The listing builds one solid part. Answer for the finished solid, in the listing's coordinates (mm). Round coordinates to 2 decimals unless told otherwise and drop trailing zeros. Order: outer loops, then holes, each group sorted by start corner. A loop starts at its lowest first (then second) coordinate and runs counter-clockwise, first axis right, second up. Notation, with made-up numbers: (37.5, 10) - (72.5, 10) arc R20 cw to (72.5, 33) - close; hole circle Ø1 at (44, -12). An arc over 180 degrees is marked (long way). Write item = value, one per line.
from build123d import *

# Parameters (mm, degrees)
SKETCH1_W                = 62
SKETCH1_H                = 60
BOSS_EXTRUDE1_DEPTH      = 3
F_4_0_4_DIAMETER_HOLE1_D = 4
FILLET1_R                = 5


with BuildPart() as part:
    # Sketch1 → Boss-Extrude1 (new body)
    with BuildSketch(Plane(origin=(0, 0, 0), x_dir=(1, 0, 0), z_dir=(0, 1, 0))):
        Rectangle(SKETCH1_W, SKETCH1_H)
    extrude(amount=BOSS_EXTRUDE1_DEPTH)

    # Ø4.0 (4) Diameter Hole1 (through all)
    with Locations(Plane(origin=(0, 3, 0), x_dir=(1, 0, 0), z_dir=(0, 1, 0))):
        with Locations((-26, 25), (26, -25), (26, 25), (-26, -25)):
            Hole(F_4_0_4_DIAMETER_HOLE1_D / 2)

    # Fillet1
    fillet1_edges = [part.edges().sort_by_distance(p)[0] for p in [
        (31, 1.5, 30),
        (-31, 1.5, 30),
        (-31, 1.5, -30),
        (31, 1.5, -30),
    ]]
    fillet(fillet1_edges, radius=FILLET1_R)


solid = part.part
Q1. Find the intervals of material crossed by line 1 (Z direction, x = 26, y = 1.2); line 2 (X direction, y = 1.85, z = 25); line 3 (X direction, y = 0.15, z = 26), in increasing order. Write a range as from..to.
Model answer:
line_1 = -30..-27, -23..23, 27..30
line_2 = -31..-28, -24..24, 28..31
line_3 = -30.9..-27.73, -24.27..24.27, 27.73..30.9
Q2. Section A-A on y = 2.4 is taken. Determine the outline of the cut face in (x, z).
Model answer:
outline = (-31, -25) arc R5 ccw to (-26, -30) - (26, -30) arc R5 ccw to (31, -25) - (31, 25) arc R5 ccw to (26, 30) - (-26, 30) arc R5 ccw to (-31, 25) - close; hole circle Ø4 at (-26, -25); hole circle Ø4 at (-26, 25); hole circle Ø4 at (26, -25); hole circle Ø4 at (26, 25)
Q3. Determine the mould class of faces 1 (the face through (31, 1, 0)), 2 (the face through (26, 1, -23)), 3 (the face through (0, 1, -30)) for opening direction X: released by +X, released by -X, zero draft, split by the parting line, or undercut.
Model answer:
face_1 = released by +X
face_2 = undercut
face_3 = zero draft
